Could you check a few things on this model? Use its own coordinates, in mm. A direction names the side the tool comes from. Give positions to 0.01 mm unless a question says otherwise; leave off trailing zeros. Write each loop counter-clockwise with the first axis right and the second up, starting at its lowest first coordinate (ties: lowest second). Pieces come first, ordered by that corner, then holes. Notation, with made-up numbers: (-10.75, 76.5) - (-1.75, 76.5) arc R14 cw to (-1.75, 88.5) - close; hole circle Ø9 at (42.25, 17). An arc over 180 degrees is marked (long way). Answer as CSV lines item,"result". Start each with the question number.
Q1. We'd pull the mould along Z, two halves only. Please class faces 3 (the face through (-19.524, 11.493, -4.336)), 4 (the face through (4, -3, 0)), 5 (the face through (0.9, 5.11, 2.86)): pulls with the +Z half, pulls with the -Z half, needs draft (parallel to the pull), parting line crosses it, or undercut.
Q2. Imagine slicing it at C-C on y = 8. List the corners of the cut face in (x, z) for me, and give its area (3 significant figures).
Q3. Imagine slicing it at A-A on x = 0. List the corners of the cut face in (y, z) for me, and give its area (3 significant figures).
Q4. Will these pins go through, and if not, where does the flat tip stop? pin 1 Ø1 at (y, z) = (6.5, 10) entering from -X; pin 2 Ø1 at (x, y) = (-12, 1) entering from +Z; pin 3 Ø2 at (x, y) = (13.5, 5) entering from +Z; pin 4 Ø5 at (x, z) = (0, 0) entering from +Y.
Q5. Imagine slicing it at B-B on z = 0. List the corners of the cut face in (x, y) for me.
Q6. On a 3-axis mill with a long thin cutter (end or side, diameter ignored), from which of +Z, -Z, +X, -X, +Y, -Y can I reach the whole of each face in a straight line? I mean faces 1 (the face through (0, 0, -16)), 2 (the face through (19.524, -1.507, -4.336)). Say none if no direction works.
Q7. If I drill on line 1 along X through (y, z) = (6.75, 0); line 2 along Y through (x, z) = (-15, -7.5); line 3 along X through (y, z) = (5.5, -1), over which ranges is the centre line in solid material (lowest first)?
```python
from build123d import *

# Parameters (mm, degrees)
SKETCH_1_R          = 15.5
EXTRUDE_1_DEPTH     = 10
SKETCH_2_R          = 20
EXTRUDE_2_DEPTH     = 3
EXTRUDE_START       = 3
SKETCH_3_R          = 20
EXTRUDE_3_DEPTH     = 3
FILLET_2_R          = 1
SKETCH_4_R          = 3
CUT_EXTRUDE_1_DEPTH = 33.49615368


with BuildPart() as part:
    # 草图1 → 凸台-拉伸1 (new body)
    with BuildSketch(Plane(origin=(0, 0, 0), x_dir=(1, 0, 0), z_dir=(0, 1, 0))):
        with Locations(Location((0, 0, 0), (0, 0, 270))):
            Circle(SKETCH_1_R)
    extrude(amount=EXTRUDE_1_DEPTH)

    # 草图2 → 凸台-拉伸2 (add)
    with BuildSketch(Plane(origin=(0, 10, 0), x_dir=(1, 0, 0), z_dir=(0, 1, 0))):
        with Locations(Location((0, 0, 0), (0, 0, 270))):
            Circle(SKETCH_2_R)
    extrude(amount=EXTRUDE_2_DEPTH)

    # 草图3 → 凸台-拉伸3 (add)
    with BuildSketch(Plane.XZ.offset(EXTRUDE_START)):
        with Locations(Location((0, 0, 0), (0, 0, 90))):
            Circle(SKETCH_3_R)
    extrude(amount=-EXTRUDE_3_DEPTH)

    # 圆角2
    fillet_2_edges = [part.edges().sort_by_distance(p)[0] for p in [
        (0, -3, -20),
        (0, 10, -20),
        (0, 13, -20),
        (0, 0, -20),
    ]]
    fillet(fillet_2_edges, radius=FILLET_2_R)

    # 草图4 → 切除-拉伸1 (cut, through all)
    with BuildSketch(Plane(origin=(0, 13, 0), x_dir=(1, 0, 0), z_dir=(0, 1, 0))):
        with Locations(Location((0, 0, 0), (0, 0, 270))):
            Circle(SKETCH_4_R)
    extrude(amount=-CUT_EXTRUDE_1_DEPTH, mode=Mode.SUBTRACT)


solid = part.part
```
Conclusion:
1,face 3,"parting line crosses it"
1,face 4,"needs draft"
1,face 5,"undercut"
2,outline,"circle Ø31 at (0, 0); hole circle Ø6 at (0, 0)"
2,area,"726 mm^2"
3,outline,"(-3, -19) arc R1 ccw to (-2, -20) - (-1, -20) arc R1 ccw to (0, -19) - (0, -15.5) - (10, -15.5) - (10, -19) arc R1 ccw to (11, -20) - (12, -20) arc R1 ccw to (13, -19) - (13, -3) - (-3, -3) - close; (-3, 3) - (13, 3) - (13, 19) arc R1 ccw to (12, 20) - (11, 20) arc R1 ccw to (10, 19) - (10, 15.5) - (0, 15.5) - (0, 19) arc R1 ccw to (-1, 20) - (-2, 20) arc R1 ccw to (-3, 19) - close"
3,area,"452 mm^2"
4,pin 1,"x = -12.25"
4,pin 2,"z = 10.39"
4,pin 3,"z = 9.17"
4,pin 4,"through"
5,outline,"(-20, -2) arc R1 ccw to (-19, -3) - (-3, -3) - (-3, 13) - (-19, 13) arc R1 ccw to (-20, 12) - (-20, 11) arc R1 ccw to (-19, 10) - (-15.5, 10) - (-15.5, 0) - (-19, 0) arc R1 ccw to (-20, -1) - close; (3, -3) - (19, -3) arc R1 ccw to (20, -2) - (20, -1) arc R1 ccw to (19, 0) - (15.5, 0) - (15.5, 10) - (19, 10) arc R1 ccw to (20, 11) - (20, 12) arc R1 ccw to (19, 13) - (3, 13) - close"
6,face 1,"none"
6,face 2,"+Y, -Y"
7,line 1,"-15.5 to -3, 3 to 15.5"
7,line 2,"-3 to 0, 10 to 13"
7,line 3,"-15.47 to -2.83, 2.83 to 15.47"
